Autodesk Inventor part; units mm, degrees
ref_plane "YZ Plane" through (0, 0, 0) normal (1, 0, 0) x (0, 1, 0)
ref_plane "XZ Plane" through (0, 0, 0) normal (0, 1, 0) x (-1, 0, 0)
ref_plane "XY Plane" through (0, 0, 0) normal (0, 0, 1) x (1, 0, 0)
sketch "Esboço1" plane through (0, 0, 0) normal (0, 0, 1) x (1, 0, 0)
  line L0 (0, 0) -> (30, 0)
  line L1 (30, 0) -> (30, -36.4)
  line L2 (30, -36.4) -> (0, -36.4)
  line L3 (0, -36.4) -> (0, 0)
  dimension "d0" = 30
  dimension "d1" = 36.4
extrude "Extrusão1" add sketch "Esboço1" along normal blind 0.5
sketch "Esboço2" plane through (0, 0, 0.5) normal (0, 0, 1) x (1, 0, 0)
  line L0 (30, 0) -> (0, 0)
  line L1 (0, 0) -> (15, 0)
  line L2 (15, 0) -> (15, -7.5)
  circle A0 centre (15, -7.5) radius 1.5
  dimension "d4" = 7.5
  dimension "d5" = 3
extrude "Extrusão2" cut sketch "Esboço2" against normal blind 0.5
sketch "Esboço4" plane through (0, 0, 0.5) normal (0, 0, 1) x (1, 0, 0)
  line L0 (0, -36.4) -> (30, -36.4)
  line L1 (0, -36.4) -> (30, -36.4)
  line L2 (30, -36.4) -> (30, -37.1)
  line L3 (30, -37.1) -> (0, -37.1)
  line L4 (0, -37.1) -> (0, -36.4)
  point P0 (0, 0)
  dimension "d10" = 0.7
extrude "Extrusão3" add sketch "Esboço4" against normal blind 0.5
sketch "Esboço5" plane through (0, 0, 0.5) normal (0, 0, 1) x (1, 0, 0)
  line L0 (0, 0) -> (0, -37.1)
  line L1 (0, -37.1) -> (4, -37.1)
  line L2 (30, -37.1) -> (0, -37.1)
  line L3 (30, -37.1) -> (30, 0)
  line L4 (30, -37.1) -> (26, -37.1)
  line L5 (30, -37.1) -> (35.5, -37.1)
  line L6 (35.5, -37.1) -> (35.5, -17.1)
  line L7 (35.5, -17.1) -> (30, -17.1)
  dimension "d13" = 4
  dimension "d14" = 4
  dimension "d15" = 5.5
  dimension "d16" = 20
extrude "Extrusão4" add sketch "Esboço5" against normal blind 0.5
sketch "Esboço6" plane through (0, 0, 0.5) normal (0, 0, 1) x (1, 0, 0)
  line L0 (35.5, -37.1) -> (0, -37.1)
  line L1 (0, -37.1) -> (9.5, -37.1)
  line L2 (35.5, -37.1) -> (31.6, -37.1)
  line L3 (35.5, -37.1) -> (36.5, -37.1)
  line L4 (36.5, -37.1) -> (36.5, -11.1125)
  line L5 (36.5, -11.1125) -> (35.5, -11.1125)
  line L6 (35.5, -11.1125) -> (35.5, -37.1)
  line L7 (30, -17.1) -> (30, 0)
  line L8 (30, -17.1) -> (30, -15.0997)
  line L9 (30, -15.0997) -> (36.5, -15.0997)
  line L10 (30, -17.1) -> (35.5, -17.1)
  line L11 (30, -17.1) -> (35.5, -17.1)
  line L12 (30, -15.0997) -> (36.5, -15.0997)
  point P0 (0, 0)
  dimension "d19" = 9.5
  dimension "d20" = 3.9
  dimension "d21" = 1
extrude "Extrusão5" add sketch "Esboço6" against normal blind 0.5 contours L6 L9 L4 L3 | L10 L7 L9 L6
sketch "Esboço7" plane through (0, 0, 0.5) normal (0, 0, 1) x (1, 0, 0)
  line L0 (36.5, -37.1) -> (0, -37.1)
  line L1 (0, -37.1) -> (9.5, -37.1)
  line L2 (36.5, -37.1) -> (31.6, -37.1)
  line L3 (31.6, -37.1) -> (31.6, -20.6)
  line L4 (9.5, -37.1) -> (9.5, -20.6)
  line L5 (8.5, -20.6) -> (8.5, -37.1)
  line L6 (32.6, -20.6) -> (32.6, -37.1)
  line L7 (31.6, -20.6) -> (31.6, -20.1)
  line L8 (31.6, -20.1) -> (32.6, -20.1)
  line L9 (32.6, -20.1) -> (32.6, -20.6375)
  line L10 (9.5, -20.6) -> (9.5, -20.1)
  line L11 (9.5, -20.1) -> (8.5, -20.1)
  line L12 (8.5, -20.1) -> (8.5, -20.8548)
  line L13 (8.5, -37.1) -> (32.6, -37.1)
  line L14 (32.6, -37.1) -> (32.6, -36.6)
  line L15 (8.5, -37.1) -> (8.5, -36.6)
  point P0 (0, 0)
  dimension "d24" = 9.5
  dimension "d25" = 4.9
  dimension "d26" = 16.5
  dimension "d27" = 1
  dimension "d28" = 1
  dimension "d29" = 0.5
  dimension "d30" = 0.5
  dimension "d31" = 0.5
extrude "Extrusão6" add sketch "Esboço7" along normal blind 12
sketch "Esboço8" plane through (0, 0, 0.5) normal (0, 0, 1) x (1, 0, 0)
  line L0 (0, 0) -> (0, -37.1)
  line L1 (0, -37.1) -> (36.5125, -37.1)
  line L2 (36.5125, -37.1) -> (36.5125, -38.1)
  line L3 (36.5125, -38.1) -> (0, -38.1)
  line L4 (0, -38.1) -> (0, -37.1)
extrude "Extrusão7" add sketch "Esboço8" against normal blind 0.5
sketch "Esboço9" plane through (0, 0, 0.5) normal (0, 0, 1) x (1, 0, 0)
  line L0 (8.5, -37.1) -> (9.5, -37.1)
  line L1 (8.5, -37.1) -> (8.5, -38.1)
  line L2 (8.5, -38.1) -> (32.6, -38.1)
  line L3 (0, -38.1) -> (36.5125, -38.1)
  line L4 (31.6, -37.1) -> (32.6, -37.1)
  line L5 (32.6, -37.1) -> (32.6, -38.1)
  line L6 (32.6165, -37.1) -> (8.5, -37.1)
  point P0 (0, 0)
extrude "Extrusão8" add sketch "Esboço9" along normal blind 12
sketch "Esboço10" plane through (0, 0, 12.5) normal (0, 0, 1) x (1, 0, 0)
  line L0 (9.5, -20.1) -> (8.5, -20.1)
  line L1 (9.5, -37.1) -> (9.5, -20.1)
  line L2 (8.5, -20.1) -> (9.5, -20.1)
  line L3 (9.5, -20.1) -> (9.5, -22.1)
  line L4 (9.5, -22.1) -> (8.5, -22.1)
  line L5 (8.5, -22.1) -> (8.5, -20.1)
  line L6 (32.6, -20.1) -> (31.6, -20.1)
  line L7 (32.6, -38.1) -> (32.6, -20.1)
  line L8 (31.6, -20.1) -> (32.6, -20.1)
  line L9 (32.6, -20.1) -> (32.6, -22.1)
  line L10 (32.6, -22.1) -> (31.6, -22.1)
  line L11 (31.6, -22.1) -> (31.6, -20.1)
  point P0 (0, 0)
  dimension "d38" = 2
extrude "Extrusão9" cut sketch "Esboço10" against normal blind 12
sketch "Esboço11" plane through (8.5, -38.1, 0.5) normal (-1, 0, 0) x (0, 0, 1)
  line L0 (12, 16) -> (0, 16)
  line L1 (12, 16) -> (12, 0)
  line L2 (0, 16) -> (12, 16)
  line L3 (12, 16) -> (12, 15.5)
  line L4 (12, 15.5) -> (0, 15.5)
  line L5 (0, 15.5) -> (0, 16)
  point P0 (-0.5, 38.1)
  dimension "d41" = 0.5
extrude "Extrusão10" add sketch "Esboço11" along normal blind 5
sketch "Esboço12" plane through (32.6, -38.1, 12.5) normal (1, 0, 0) x (0, 0, -1)
  line L0 (12, 16) -> (0, 16)
  line L1 (12, 15.5) -> (0, 15.5)
  line L2 (0, 16) -> (12, 16)
  line L3 (12, 16) -> (12, 15.5)
  line L4 (12, 15.5) -> (0, 15.5)
  line L5 (0, 15.5) -> (0, 16)
  point P0 (12.5, 38.1)
extrude "Extrusão11" add sketch "Esboço12" along normal blind 5
sketch "Esboço13" plane through (0, 0, 0.5) normal (0, 0, 1) x (1, 0, 0)
  circle A0 centre (15, -7.5) radius 1.5
  line L0 (15, -7.5) -> (30, -7.5)
  line L1 (30, -15.0997) -> (30, 0)
  line L2 (15, -7.5) -> (0, -7.5)
  line L3 (0, -38.1) -> (0, 0)
  line L4 (0, 0) -> (30, 0)
  line L5 (30, 0) -> (0, 0)
  line L6 (30, 0) -> (30, -7.5)
  line L7 (0, -7.5) -> (0, 0)
  point P0 (13.5, -7.5)
  point P1 (16.5, -7.5)
extrude "Extrusão12" cut sketch "Esboço13" against normal blind 5 contours A0 L2 L3 L4 L1 L0
sketch "Esboço14" plane through (31.6, -22.1, 12.5) normal (0, 1, 0) x (1, 0, 0)
  line L0 (-22.1, 0) -> (-28.1, 0)
  line L1 (-28.1, 0) -> (-25.1, 0)
  line L2 (-25.1, 0) -> (-25.1, 6)
  line L3 (-22.1, 12) -> (-28.1, 12)
  line L4 (6, 12) -> (6, 0)
  line L5 (6, 0) -> (3, 0)
  line L6 (6, 0) -> (0, 0)
  line L7 (3, 0) -> (3, 6)
  circle A0 centre (-25.1, 6) radius 0.5
  circle A1 centre (3, 6) radius 0.5
  point P0 (-31.6, 12.5)
  dimension "d48" = 6
  dimension "d49" = 1
  dimension "d50" = 1
extrude "Extrusão13" cut sketch "Esboço14" against normal blind 5
sketch "Esboço15" plane through (37.6, -22.1, 0.5) normal (0, 0, -1) x (-1, 0, 0)
  line L0 (7.6, 7.0003) -> (1.1, 7.0003)
  line L1 (1.1, 7.0003) -> (0, 7.0003)
  line L2 (0, 7.0003) -> (0, -16)
  line L3 (1.0875, -15) -> (1.0875, -16)
  line L4 (0, -16) -> (1.0875, -16)
  line L5 (1.1, 7.0003) -> (1.8775, 7.0003)
  line L6 (1.8775, 7.0003) -> (1.8775, -16)
  line L7 (1.0875, -16) -> (37.6, -16)
  line L8 (0, -16) -> (1.8775, -16)
  point P0 (37.6, 22.1)
extrude "Extrusão14" add sketch "Esboço15" along normal blind 0.5
properties part number "tampa"
Read the model definition and answer for the solid it produces. Units are mm, in the model's axes. A direction names the side the tool comes from. Coordinates: 2 decimals unless noted, no trailing zeros. Write each loop counter-clockwise with the first axis right and the second up, starting at its lowest first coordinate (ties: lowest second). Pieces come first, ordered by that corner, then holes. Notation, with made-up numbers: (-23.5, 21) -> (18.5, 21) arc R26 ccw to (18.5, 35) -> close; hole circle Ø2 at (83, 38). An arc over 180 degrees is marked (long way). Write item = value, one per line.
(1) Section D-D on x = 6.5 is taken. Write down the section's boundary in (y, z), plus the area to 3 significant figures.
From the geometry:
outline = (-38.1, 0) -> (-7.5, 0) -> (-7.5, 0.5) -> (-22.1, 0.5) -> (-22.1, 6) -> (-22.6, 6) -> (-22.6, 0.5) -> (-38.1, 0.5) -> close; (-22.6, 7) -> (-22.1, 7) -> (-22.1, 12.5) -> (-22.6, 12.5) -> close
area = 20.8 mm2
(2) Section B-B on z = 6.5 is taken. Write down the section's boundary in (x, y), plus the area to 3 significant figures.
From the geometry:
outline = (3.5, -22.6) -> (6, -22.6) -> (6, -22.1) -> (3.5, -22.1) -> close; (7, -22.6) -> (8.5, -22.6) -> (8.5, -38.1) -> (32.6, -38.1) -> (32.6, -22.6) -> (34.1, -22.6) -> (34.1, -22.1) -> (31.6, -22.1) -> (31.6, -37.1) -> (9.5, -37.1) -> (9.5, -22.1) -> (7, -22.1) -> close; (35.1, -22.6) -> (37.6, -22.6) -> (37.6, -22.1) -> (35.1, -22.1) -> close
area = 58.1 mm2
(3) Straight lines are drawn through the part: L1, parallel to X at y = -22.35, z = 6.5; L2, parallel to X at y = -23, z = 7; L3, parallel to Z at x = 34.6, y = -22.3. For each, find the intervals that lie inside material, in ascending order. Write a range as from..to.
From the geometry:
L1 = 3.5..6, 7..9.5, 31.6..34.1, 35.1..37.6
L2 = 8.5..9.5, 31.6..32.6
L3 = 0..6, 7..12.5
(4) Section A-A on x = 34.6 is taken. Write down the section's boundary in (y, z), plus the area to 3 significant figures.
From the geometry:
outline = (-38.1, 0) -> (-15.1, 0) -> (-15.1, 0.5) -> (-22.1, 0.5) -> (-22.1, 6) -> (-22.6, 6) -> (-22.6, 0.5) -> (-38.1, 0.5) -> close; (-22.6, 7) -> (-22.1, 7) -> (-22.1, 12.5) -> (-22.6, 12.5) -> close
area = 17.0 mm2
(5) Section C-C on z = 4.5 is taken. Write down the section's boundary in (x, y).
From the geometry:
outline = (3.5, -22.6) -> (8.5, -22.6) -> (8.5, -38.1) -> (32.6, -38.1) -> (32.6, -22.6) -> (37.6, -22.6) -> (37.6, -22.1) -> (31.6, -22.1) -> (31.6, -37.1) -> (9.5, -37.1) -> (9.5, -22.1) -> (3.5, -22.1) -> close
(6) Which of the six approach directions +Z, -Z, +X, -X, +Y, -Y give full straight-line access (tool end or side, diameter ignored) to faces 4 (the face through (36, -22.6, 6)), 5 (the face through (6, -22.1, 7)), 6 (the face through (8.5, -30, 6)), 7 (the face through (21, -37.1, 6))?
From the geometry:
face_4 = +Z, +X, -Y
face_5 = +Z, +X, -X, +Y
face_6 = +Z, -X, -Y
face_7 = +Z, +Y
(7) For a pull along Z with two mould halves and no side action, classify faces 1 (the face through (6.392, -22.347, 6.988)), 2 (the face through (19, -23, 0)), 3 (the face through (34, -22.1, 6)) as +Z half, -Z half, draft (parallel to the pull), parting line (faces both ways), or undercut.
From the geometry:
face_1 = undercut
face_2 = -Z half
face_3 = draft
(8) Given pin 1 Ø1 at (x, z) = (27, 6) entering from +Y; pin 2 Ø2.5 at (x, y) = (36, -27.5) entering from +Z; pin 3 Ø6 at (y, z) = (-27.5, 8) entering from +X; pin 4 Ø5 at (x, y) = (4.5, -25) entering from +Z, each flat-ended and moving along its own axis, determine where each tip first touches the part or whether it passes through.
From the geometry:
pin_1 = -37.1
pin_2 = 0.5
pin_3 = 32.6
pin_4 = 12.5
